Verification items for the finished model (mm, model axes). Give positions to 0.01 mm unless a question says otherwise; leave off trailing zeros. Loops run counter-clockwise (first coordinate to the right, second up) from the corner with the lowest first, then second, coordinate; pieces in that order, holes last. Notation, with made-up numbers: (-38.75, 66.5) - (-24.75, 66.5) arc R13 ccw to (-24.75, 71.5) - close; hole circle Ø10 at (70.25, -20). An arc over 180 degrees is marked (long way). One line per item, written item: value. Start each with the question number.
1. Sectioned sample at A-A (y = 55). Record the cut outline in (x, z), plus the area to 3 significant figures.
2. Scan lines: L1, parallel to X at y = 55, z = 2.45; L2, parallel to Y at x = -58.5, z = 2. Record each from-to range of solid material in increasing order. Write a range as [from, to].
3. Sectioned sample at C-C (x = -62.5). Record the cut outline in (y, z).
4. Gauge pin test, flat ends, axial feed: pin 1 (0.8 mm diameter, centred on y = 25, z = 2, fed in from -X); pin 2 (2 mm diameter, centred on x = -38, y = 22.5, fed in from -Z); pin 3 (0.8 mm diameter, centred on y = 36.5, z = 2, fed in from +X); pin 4 (0.8 mm diameter, centred on x = -143.5, z = 1, fed in from +Y). Record the tip position at first contact, or that the pin passes through.
5. Sectioned sample at B-B (z = 1.1). Record the cut outline in (x, y).
Autodesk Inventor part; units mm, degrees
ref_plane "YZ Plane" through (0, 0, 0) normal (1, 0, 0) x (0, 1, 0)
ref_plane "XZ Plane" through (0, 0, 0) normal (0, 1, 0) x (-1, 0, 0)
ref_plane "XY Plane" through (0, 0, 0) normal (0, 0, 1) x (1, 0, 0)
sketch "Sketch1" plane through (0, 0, 0) normal (0, 0, 1) x (1, 0, 0)
  line L0 (-149.3708, -1.27) -> (-22.3708, -1.27)
  line L1 (-22.3708, -1.27) -> (-22.3708, 1.27)
  line L2 (-149.3708, 1.27) -> (-149.3708, -1.27)
  line L3 (-149.3708, -1.27) -> (-22.3708, 1.27) construction
  line L4 (-22.3708, -1.27) -> (-149.3708, 1.27) construction
  line L5 (-149.3708, 1.27) -> (-136.6708, 1.27)
  line L6 (-22.3708, 1.27) -> (-35.0708, 1.27)
  line L7 (-130.3208, 1.27) -> (-130.3208, 77.47)
  line L8 (-130.3208, 77.47) -> (-136.6708, 77.47)
  line L9 (-136.6708, 77.47) -> (-136.6708, 1.27)
  line L10 (-130.3208, 1.27) -> (-104.9208, 1.27)
  line L11 (-98.5708, 1.27) -> (-98.5708, 77.47)
  line L12 (-98.5708, 77.47) -> (-104.9208, 77.47)
  line L13 (-104.9208, 77.47) -> (-104.9208, 1.27)
  line L14 (-41.4208, 1.27) -> (-41.4208, 77.47)
  line L15 (-41.4208, 77.47) -> (-35.0708, 77.47)
  line L16 (-35.0708, 77.47) -> (-35.0708, 1.27)
  line L17 (-41.4208, 1.27) -> (-66.8208, 1.27)
  line L18 (-73.1708, 1.27) -> (-73.1708, 77.47)
  line L19 (-73.1708, 77.47) -> (-66.8208, 77.47)
  line L20 (-66.8208, 77.47) -> (-66.8208, 1.27)
  line L21 (-98.5708, 1.27) -> (-73.1708, 1.27)
  point P0 (0, 0)
  point P1 (-85.8708, 0)
  dimension "d0" = 127
  dimension "d1" = 2.54
  dimension "d2" = 12.7
  dimension "d3" = 12.7
  dimension "d4" = 6.35
  dimension "d5" = 76.2
  dimension "d6" = 25.4
  dimension "d7" = 6.35
  dimension "d8" = 6.35
  dimension "d9" = 76.2
  dimension "d10" = 25.4
  dimension "d11" = 6.35
  dimension "d12" = 76.2
extrude "Extrusion1" add sketch "Sketch1" along normal blind 2.54
properties part number "Bucket - Rake"
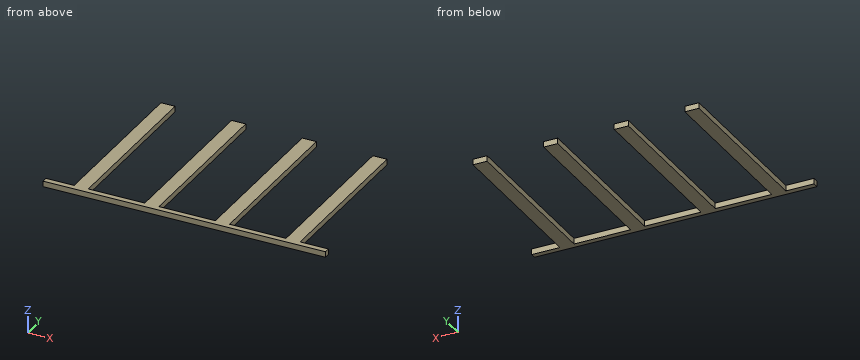
Results are:
1. outline: (-136.67, 0) - (-130.32, 0) - (-130.32, 2.54) - (-136.67, 2.54) - close; (-104.92, 0) - (-98.57, 0) - (-98.57, 2.54) - (-104.92, 2.54) - close; (-73.17, 0) - (-66.82, 0) - (-66.82, 2.54) - (-73.17, 2.54) - close; (-41.42, 0) - (-35.07, 0) - (-35.07, 2.54) - (-41.42, 2.54) - close
1. area: 64.5 mm^2
2. L1: x = [-136.67, -130.32], [-104.92, -98.57], [-73.17, -66.82], [-41.42, -35.07]
2. L2: y = [-1.27, 1.27]
3. outline: (-1.27, 0) - (1.27, 0) - (1.27, 2.54) - (-1.27, 2.54) - close
4. pin 1: stops at x = -136.67
4. pin 2: stops at z = 0
4. pin 3: stops at x = -35.07
4. pin 4: stops at y = 1.27
5. outline: (-149.37, -1.27) - (-22.37, -1.27) - (-22.37, 1.27) - (-35.07, 1.27) - (-35.07, 77.47) - (-41.42, 77.47) - (-41.42, 1.27) - (-66.82, 1.27) - (-66.82, 77.47) - (-73.17, 77.47) - (-73.17, 1.27) - (-98.57, 1.27) - (-98.57, 77.47) - (-104.92, 77.47) - (-104.92, 1.27) - (-130.32, 1.27) - (-130.32, 77.47) - (-136.67, 77.47) - (-136.67, 1.27) - (-149.37, 1.27) - close
